Check sheet for the modelled part. Datum: model origin and axes. Units: mm. A direction names the side the tool comes from. Round coordinates to 2 decimals unless told otherwise and drop trailing zeros. Write each loop counter-clockwise with the first axis right and the second up, starting at its lowest first coordinate (ties: lowest second). Pieces come first, ordered by that corner, then holes.
from build123d import *

# Parameters (mm, degrees)
BOSS_EXTRU_1_DEPTH      = 37.5
BOSS_EXTRU_2_DEPTH      = 4
ESQUISSE3_R             = 2
ENL_V_MAT_EXTRU_1_DEPTH = 56.418859606
ESQUISSE5_R             = 3
ENL_V_MAT_EXTRU_2_DEPTH = 4
CONG_1_R                = 7
CONG_2_R                = 3


with BuildPart() as part:
    # Esquisse1 → Boss.-Extru.1 (new body)
    with BuildSketch(Plane(origin=(0, 0, 0), x_dir=(1, 0, 0), z_dir=(0, 1, 0))):
        with BuildLine():
            Line((0, 29.133924434), (0, 39))
            Line((0, 39), (12, 39))
            Line((12, 39), (12, 0))
            Line((12, 0), (0, 0))
            Line((0, 0), (0, 9.866075566))
            ThreePointArc((0, 9.866075566), (8.25, 19.5), (0, 29.133924434))
        make_face()
    extrude(amount=BOSS_EXTRU_1_DEPTH)

    # Esquisse2 → Boss.-Extru.2 (add)
    with BuildSketch(Plane.XZ):
        with BuildLine():
            Line((0, 0), (12, 0))
            Line((12, 0), (12, -39))
            Line((12, -39), (0, -39))
            Line((0, -39), (0, -26.848469228))
            ThreePointArc((0, -26.848469228), (6, -19.5), (0, -12.151530772))
            Line((0, -12.151530772), (0, 0))
        make_face()
    boss_extru_2 = extrude(amount=-BOSS_EXTRU_2_DEPTH)

    # Symétrie1: Boss.-Extru.2 across plane
    add(boss_extru_2.mirror(Plane.ZX.offset(18.75)))

    # Esquisse3 → Enlèv. mat.-Extru.1 (cut, through all)
    with BuildSketch(Plane.ZY):
        with Locations((-34.066962217, 33.5)):
            Circle(ESQUISSE3_R)
        with Locations(Location((-34.066962217, 4, 0), (0, 0, 180))):
            Circle(ESQUISSE3_R)
        with Locations((-4.933037783, 4)):
            Circle(ESQUISSE3_R)
        with Locations(Location((-4.933037783, 33.5, 0), (0, 0, 180))):
            Circle(ESQUISSE3_R)
    extrude(amount=-ENL_V_MAT_EXTRU_1_DEPTH, mode=Mode.SUBTRACT)

    # Esquisse5 → Enlèv. mat.-Extru.2 (cut)
    with BuildSketch(Plane(origin=(12, 0, 0), x_dir=(0, 0, -1), z_dir=(1, 0, 0))):
        with Locations((4.933037783, 33.5)):
            Circle(ESQUISSE5_R)
        with Locations((34.066962217, 33.5)):
            Circle(ESQUISSE5_R)
        with Locations((34.066962217, 4)):
            Circle(ESQUISSE5_R)
        with Locations((4.933037783, 4)):
            Circle(ESQUISSE5_R)
    extrude(amount=-ENL_V_MAT_EXTRU_2_DEPTH, mode=Mode.SUBTRACT)

    # Congé1
    # the kernel refuses this fillet: 7 mm, written as the material it takes off along each edge
    with BuildSketch(Plane(origin=(12, 55, -39), x_dir=(-1, 0, 0), z_dir=(0, -1, 0)), Plane(origin=(12, 55, 0), x_dir=(0, 0, -1), z_dir=(0, -1, 0))) as cong_1_piece_1:
        with BuildLine():
            CenterArc((CONG_1_R, -CONG_1_R), CONG_1_R, 90, 90)
            Line((0, -CONG_1_R), (0, 0))
            Line((0, 0), (CONG_1_R, 0))
        make_face()
    extrude(amount=72.5, mode=Mode.SUBTRACT)

    # Congé2
    # the kernel refuses this fillet: 3 mm, written as the material it takes off along each edge
    with BuildSketch(Plane(origin=(5, 0, 0), x_dir=(0, 0, -1), z_dir=(-1, 0, 0)), Plane(origin=(-7.5, 0, -39), x_dir=(0, 0, 1), z_dir=(1, 0, 0)), Plane(origin=(-7.5, 37.5, -39), x_dir=(0, -1, 0), z_dir=(1, 0, 0))) as cong_2_piece_1:
        with BuildLine():
            CenterArc((CONG_2_R, -CONG_2_R), CONG_2_R, 90, 90)
            Line((0, -CONG_2_R), (0, 0))
            Line((0, 0), (CONG_2_R, 0))
        make_face()
    extrude(amount=12.5, mode=Mode.SUBTRACT)
    with BuildSketch(Plane(origin=(5, 0, -7), x_dir=(0, 0, 1), z_dir=(-1, 0, 0))) as cong_2_piece_2:
        with BuildLine():
            CenterArc((7 - CONG_2_R, CONG_2_R), CONG_2_R, 270, 90)
            Line((7, CONG_2_R), (7, 0))
            Line((7, 0), (7 - CONG_2_R, 0))
        make_face()
    revolve(axis=Axis((5, 0, -7), (0, 1, 0)), revolution_arc=90, mode=Mode.SUBTRACT)
    with BuildSketch(Plane(origin=(5, 0, -32), x_dir=(1, 0, 0), z_dir=(0, 0, 1))) as cong_2_piece_3:
        with BuildLine():
            CenterArc((7 - CONG_2_R, CONG_2_R), CONG_2_R, 270, 90)
            Line((7, CONG_2_R), (7, 0))
            Line((7, 0), (7 - CONG_2_R, 0))
        make_face()
    revolve(axis=Axis((5, 0, -32), (0, 1, 0)), revolution_arc=90, mode=Mode.SUBTRACT)
    with BuildSketch(Plane(origin=(5, 37.5, 0), x_dir=(0, 0, -1), z_dir=(-1, 0, 0))) as cong_2_piece_4:
        with BuildLine():
            CenterArc((CONG_2_R, CONG_2_R), CONG_2_R, 180, 90)
            Line((0, CONG_2_R), (0, 0))
            Line((0, 0), (CONG_2_R, 0))
        make_face()
    extrude(amount=12.5, mode=Mode.SUBTRACT)
    with BuildSketch(Plane(origin=(5, 37.5, -7), x_dir=(0, 0, 1), z_dir=(-1, 0, 0))) as cong_2_piece_5:
        with BuildLine():
            CenterArc((7 - CONG_2_R, -CONG_2_R), CONG_2_R, 0, 90)
            Line((7, -CONG_2_R), (7, 0))
            Line((7, 0), (7 - CONG_2_R, 0))
        make_face()
    revolve(axis=Axis((5, 37.5, -7), (0, 1, 0)), revolution_arc=90, mode=Mode.SUBTRACT)
    with BuildSketch(Plane(origin=(5, 37.5, -32), x_dir=(1, 0, 0), z_dir=(0, 0, 1))) as cong_2_piece_6:
        with BuildLine():
            CenterArc((7 - CONG_2_R, -CONG_2_R), CONG_2_R, 0, 90)
            Line((7, -CONG_2_R), (7, 0))
            Line((7, 0), (7 - CONG_2_R, 0))
        make_face()
    revolve(axis=Axis((5, 37.5, -32), (0, 1, 0)), revolution_arc=90, mode=Mode.SUBTRACT)
    with BuildSketch(Plane(origin=(12, 0, -32), x_dir=(-1, 0, 0), z_dir=(0, 0, 1))) as cong_2_piece_7:
        with BuildLine():
            CenterArc((CONG_2_R, -CONG_2_R), CONG_2_R, 90, 90)
            Line((0, -CONG_2_R), (0, 0))
            Line((0, 0), (CONG_2_R, 0))
        make_face()
    extrude(amount=25, mode=Mode.SUBTRACT)
    with BuildSketch(Plane(origin=(12, 37.5, -32), x_dir=(-1, 0, 0), z_dir=(0, 0, 1))) as cong_2_piece_8:
        with BuildLine():
            CenterArc((CONG_2_R, CONG_2_R), CONG_2_R, 180, 90)
            Line((0, CONG_2_R), (0, 0))
            Line((0, 0), (CONG_2_R, 0))
        make_face()
    extrude(amount=25, mode=Mode.SUBTRACT)


solid = part.part
1. Set-up check for faces 5 (the flat face through (8, 36, -5)), 6 (the cylindrical face through (3.944, 31.548, -34.501)), 7 (the cylindrical face through (8.25, 18.54, -19.31)): record each of +Z, -Z, +X, -X, +Y, -Y from which the full face is reachable in a straight line by a thin tool's end or side.
2. Sectioned sample at A-A, the plane x = 2.5. Enter the section's corners in (y, z), plus the area to 3 significant figures.
3. Release check for a two-part mould opening along Z. For faces 1 (the cylindrical face through (11.1, 0.86, -19.68)), 2 (the cylindrical face through (6, 2, -19.6)), 3 (the cylindrical face through (9.58, 33.63, -31.07)), 4 (the flat face through (2, 19, -39)) record: released by +Z, released by -Z, zero draft, split by the parting line, or undercut.
4. Sectioned sample at C-C, the plane y = 26. Enter the section's corners in (x, z).
5. Sectioned sample at D-D, the plane z = -28. Enter the section's corners in (x, y).
6. Sectioned sample at B-B, the plane y = 4.5. Enter the section's corners in (x, z) (3 decimals), plus the area to 3 significant figures.
7. Go/stop test with flat-tipped pins: pin 1 (3 mm diameter, centred on x = 10, y = 30.5, fed in from +Z); pin 2 (5 mm diameter, centred on y = 33.5, z = -4.93, fed in from +X). Record where each tip stops, or that it passes through.
8. Scan lines: line 1 along Y through (x, z) = (5.25, -5); line 2 along Y through (x, z) = (7.25, -5.5); line 3 along Y through (x, z) = (7.75, -18). Record each from-to range of solid material in increasing order.
Computed values:
1. face 5: +X
1. face 6: +X, -X
1. face 7: -X
2. outline: (0, -36) arc R3 ccw to (3, -39) - (34.5, -39) arc R3 ccw to (37.5, -36) - (37.5, -25.84) - (33.5, -25.84) - (33.5, -28.39) - (4, -28.39) - (4, -25.84) - (0, -25.84) - close; (0, -13.16) - (4, -13.16) - (4, -10.61) - (33.5, -10.61) - (33.5, -13.16) - (37.5, -13.16) - (37.5, -3) arc R3 ccw to (34.5, 0) - (3, 0) arc R3 ccw to (0, -3) - close; hole circle Ø4 at (4, -34.07); hole circle Ø4 at (4, -4.93); hole circle Ø4 at (33.5, -34.07); hole circle Ø4 at (33.5, -4.93)
2. area: 778 mm2
3. face 1: zero draft
3. face 2: undercut
3. face 3: undercut
3. face 4: released by -Z
4. outline: (0, -39) - (5, -39) arc R7 ccw to (12, -32) - (12, -7) arc R7 ccw to (5, 0) - (0, 0) - (0, -9.87) arc R9.75 cw to (0, -29.13) - close
5. outline: (0, 0) - (9, 0) arc R3 ccw to (12, 3) - (12, 34.5) arc R3 ccw to (9, 37.5) - (0, 37.5) - (0, 33.5) - (3.28, 33.5) - (3.28, 4) - (0, 4) - close
6. outline: (0, -39) - (5, -39) arc R7 ccw to (9.873, -37.025) - (8, -37.025) - (8, -36.003) - (0, -36.003) - close; (0, -32.13) - (8, -32.13) - (8, -31.109) - (12, -31.109) - (12, -7.891) - (8, -7.891) - (8, -6.87) - (0, -6.87) - (0, -9.866) arc R9.75 cw to (0, -29.134) - close; (0, -2.997) - (8, -2.997) - (8, -1.975) - (9.873, -1.975) arc R7 ccw to (5, 0) - (0, 0) - close
6. area: 224 mm2
7. pin 1: stops at z = -0.94
7. pin 2: stops at x = 8
8. line 1: y = 0 to 2, 6 to 31.5, 35.5 to 37.5
8. line 2: y = 0 to 2.08, 5.92 to 31.58, 35.42 to 37.5
8. line 3: y = 0 to 4, 33.5 to 37.5
